The listing builds one solid part. Answer for the finished solid, in the listing's coordinates (mm). A direction names the side the tool comes from. Coordinates: 2 decimals unless noted, no trailing zeros. Order: outer loops, then holes, each group sorted by start corner. A loop starts at its lowest first (then second) coordinate and runs counter-clockwise, first axis right, second up.
from build123d import *

# Parameters (mm, degrees)
SKETCH1_R               = 50
BOSS_EXTRUDE1_DEPTH     = 50
BOSS_EXTRUDE1_TAPER     = 20
CUT_EXTRUDE1_DEPTH      = 123.474487302
CUT_EXTRUDE1_DEPTH_BACK = 123.474487302
SKETCH2_R               = 25
SKETCH3_R               = 35
CUT_EXTRUDE2_DEPTH      = 10
CUT_EXTRUDE5_START      = -10
SKETCH5_R               = 35
CUT_EXTRUDE5_DEPTH      = 10
FILLET1_R               = 25
CUT_EXTRUDE6_DEPTH      = 123.474487302
CUT_EXTRUDE6_DEPTH_BACK = 123.474487302


with BuildPart() as part:
    # Sketch1 → Boss-Extrude1 (new body)
    with BuildSketch(Plane(origin=(0, 0, 0), x_dir=(1, 0, 0), z_dir=(0, 1, 0))):
        Circle(SKETCH1_R)
    boss_extrude1 = extrude(amount=BOSS_EXTRUDE1_DEPTH, taper=BOSS_EXTRUDE1_TAPER)

    # Mirror2: Boss-Extrude1 across plane
    add(boss_extrude1.mirror(Plane.ZX.offset(50)))

    # Sketch2 → Cut-Extrude1 (cut, two sides: drawn at the far end of the back side and taken through both)
    with BuildSketch(Plane(origin=(0, 100, 0), x_dir=(1, 0, 0), z_dir=(0, 1, 0)).offset(-CUT_EXTRUDE1_DEPTH_BACK)):
        with Locations(Location((0, 0, 0), (0, 0, 270))):
            Circle(SKETCH2_R)
    extrude(amount=CUT_EXTRUDE1_DEPTH + CUT_EXTRUDE1_DEPTH_BACK, mode=Mode.SUBTRACT)

    # Sketch3 → Cut-Extrude2 (cut)
    with BuildSketch(Plane(origin=(0, 100, 0), x_dir=(1, 0, 0), z_dir=(0, 1, 0))):
        with Locations(Location((0, 0, 0), (0, 0, 270))):
            Circle(SKETCH3_R)
    extrude(amount=-CUT_EXTRUDE2_DEPTH, mode=Mode.SUBTRACT)

    # Sketch5 → Cut-Extrude5 (cut)
    with BuildSketch(Plane.XZ.offset(CUT_EXTRUDE5_START)):
        with Locations(Location((0, 0, 0), (0, 0, 90))):
            Circle(SKETCH5_R)
    extrude(amount=CUT_EXTRUDE5_DEPTH, mode=Mode.SUBTRACT)

    # Fillet1
    fillet1_edges = [part.edges().sort_by_distance(p)[0] for p in [
        (-31.801488287, 50, 0),
    ]]
    fillet(fillet1_edges, radius=FILLET1_R)

    # Sketch7 → Cut-Extrude6 (cut, two sides: drawn at the far end of the back side and taken through both)
    with BuildSketch(Plane(origin=(0, 100, 0), x_dir=(1, 0, 0), z_dir=(0, 1, 0)).offset(-CUT_EXTRUDE6_DEPTH_BACK)):
        with BuildLine():
            Line((0, -50), (0, 0))
            Line((0, 0), (50, 0))
            ThreePointArc((50, 0), (35.355339059, -35.355339059), (0, -50))
        make_face()
    extrude(amount=CUT_EXTRUDE6_DEPTH + CUT_EXTRUDE6_DEPTH_BACK, mode=Mode.SUBTRACT)


solid = part.part
1) A tool of negligible diameter and unlimited length cuts with its end or side. For faces 4 (the face through (-26.65, 30.23, -28.47)), 5 (the face through (-25.55, 5.07, -23.92)), 6 (the face through (-23.92, 95.07, -25.55)), from which of +Z, -Z, +X, -X, +Y, -Y can it reach the whole face along a straight path? Write none if from no direction.
2) Section B-B (y = 38) is taken. Give the vertices of the cut face in (x, z), then the cut area to 3 significant figures.
3) Section A-A (y = 26) is taken. Give the vertices of the cut face in (x, z).
4) Consider L1, parallel to X at y = 30.5, z = -20.5; L2, parallel to Y at x = -25.5, z = -38; L3, parallel to X at y = 24.5, z = -2. Determine where each line is inside the solid, lowest interval first.
5) Determine the mould class of faces 1 (the face through (32, 49, 0)), 2 (the face through (0, 49, 32)), 3 (the face through (-18, 90, -18)) for opening direction X: released by +X, released by -X, zero draft, split by the parting line, or undercut.
6) Each of these flat-tipped pins is pushed along its axis until it touches: P1, Ø1, axis at y = 33.5, z = 7.5, coming from the +X side; P2, Ø21, axis at x = 9.5, z = 8, coming from the +Y side; P3, Ø8, axis at x = 14, z = -21.5, coming from the -Y side; P4, Ø1, axis at x = -18, y = 34.5, coming from the -Z side. Where does it stop, or does it pass through?
Filled sheet:
1. face 4: none
1. face 5: -Y
1. face 6: +Y
2. outline: (0, 25) - (0, 36.17) arc R36.17 ccw (long way) to (36.17, 0) - (25, 0) arc R25 cw (long way) to start
2. area: 1,610 mm2
3. outline: (0, 25) - (0, 40.54) arc R40.54 ccw (long way) to (40.54, 0) - (25, 0) arc R25 cw (long way) to start
4. L1: x = -33.06 to -14.31, 14.31 to 33.06
4. L2: y = 0 to 11.64, 88.36 to 100
4. L3: x = -41.03 to -24.92, 24.92 to 41.03
5. face 1: zero draft
5. face 2: released by +X
5. face 3: undercut
6. P1: stops at x = -23.69
6. P2: passes through
6. P3: stops at y = 10
6. P4: stops at z = -33.17
